```python
from build123d import *

# Parameters (mm, degrees)
SKETCH1_R           = 25
BOSS_EXTRUDE1_DEPTH = 40
CUT_EXTRUDE1_START  = -8
CUT_EXTRUDE1_DEPTH  = 8
CIRPATTERN1_COUNT   = 3
SKETCH7_R           = 15.1
CUT_EXTRUDE3_DEPTH  = 8.7
SKETCH8_R           = 1.5
CUT_EXTRUDE4_DEPTH  = 48.219593391


with BuildPart() as part:
    # Sketch1 → Boss-Extrude1 (new body)
    with BuildSketch(Plane(origin=(0, 0, 0), x_dir=(1, 0, 0), z_dir=(0, 1, 0))):
        with Locations(Location((0, 0, 0), (0, 0, 270))):
            Circle(SKETCH1_R)
    extrude(amount=BOSS_EXTRUDE1_DEPTH)

    # Sketch2 → Cut-Extrude1 (cut)
    with BuildSketch(Plane(origin=(0, 40, 0), x_dir=(1, 0, 0), z_dir=(0, 1, 0)).offset(CUT_EXTRUDE1_START)):
        with BuildLine():
            Line((-25, 0), (-5, 0))
            Line((-5, 0), (-5, -16.4))
            Line((-5, -16.4), (-13.2, -16.4))
            Line((-13.2, -16.4), (-13.2, -8.2))
            Line((-13.2, -8.2), (-23.616943071, -8.2))
            ThreePointArc((-23.616943071, -8.2), (-24.651811057, -4.157909525), (-25, 0))
        make_face()
    cut_extrude1 = extrude(amount=CUT_EXTRUDE1_DEPTH, mode=Mode.SUBTRACT)

    # CirPattern1: Cut-Extrude1 ×3 about axis
    cirpattern1_axis = Axis((0, 0, 0), (0, 1, 0))
    for i in range(1, CIRPATTERN1_COUNT):
        add(cut_extrude1.rotate(cirpattern1_axis, i * 360 / CIRPATTERN1_COUNT), mode=Mode.SUBTRACT)

    # Sketch7 → Cut-Extrude3 (cut)
    with BuildSketch(Plane.XZ):
        with Locations(Location((0, 0, 0), (0, 0, 270))):
            Circle(SKETCH7_R)
    extrude(amount=-CUT_EXTRUDE3_DEPTH, mode=Mode.SUBTRACT)

    # Sketch8 → Cut-Extrude4 (cut, through all)
    with BuildSketch(Plane.XZ.offset(-8.7)):
        with Locations(Location((0, 0, 0), (0, 0, 270))):
            Circle(SKETCH8_R)
    extrude(amount=-CUT_EXTRUDE4_DEPTH, mode=Mode.SUBTRACT)


solid = part.part
```
Here's how the part is built. I have some questions about the finished solid (model axes, mm). A direction names the side the tool comes from. Give positions to 0.01 mm unless a question says otherwise; leave off trailing zeros. Loops run counter-clockwise (first coordinate to the right, second up) from the corner with the lowest first, then second, coordinate; pieces in that order, holes last. Notation, with made-up numbers: M -22,63.25 L -17,63.25 A19 ccw -17,68.25 Z; hole C 68.25,52 d4. An arc over 180 degrees is marked long. Use one line per item in the form item = value. Start each with the question number.
Q1. Which directions (+Z, -Z, +X, -X, +Y, -Y) give clear straight access to the entire face, cutting with the end or side of a thin tool? Please do faces 5 (the flat face through (-18, 36, 8.2)), 6 (the flat face through (16.27, 35.94, 11.78)), 7 (the flat face through (0, 8.7, -3)), 8 (the flat face through (-9.7, 35.9, -16)).
Q2. If we section it at A-A (x = 10.5): Write out the boundary of the cut face in (y, z).
Q3. I need wall thicknesses on line 1 along X through (y, z) = (24, 0); line 2 along X through (y, z) = (5, 0); line 3 along Z through (x, y) = (0.5, 8.5) (3 decimals). Which ranges of each line are inside material? Lowest first, please.
Q4. If we section it at D-D (x = 20): Write out the boundary of the cut face in (y, z).
Q5. Will these pins go through, and if not, where does the flat tip stop? pin 1 Ø6 at (x, y) = (-15.5, 14.5) entering from +Z; pin 2 Ø6.5 at (y, z) = (37.5, 11.5) entering from +X; pin 3 Ø1.5 at (y, z) = (19, 2) entering from -X.
Q6. If we section it at B-B (y = 4): Write out the boundary of the cut face in (x, z), then the cut area to 3 significant figures.
Q7. Thinking about a two-plate mould opening in Z: for faces 1 (the cylindrical face through (7.509, 19.72, 23.846)), 2 (the flat face through (18.724, 35.944, -0.369)), 3 (the flat face through (-11, 0, 11)), 4 (the flat face through (2.066, 35.944, -19.979)), which applies, +Z half, -Z half, draft (parallel to the pull), parting line (faces both ways), or undercut?
Q8. If we section it at C-C (z = -14): Write out the boundary of the cut face in (x, y).
Taken from the geometry:
q1.face_5 = -X, +Y
q1.face_6 = +Z, +Y
q1.face_7 = -Y
q1.face_8 = +Y
q2.outline = M 0,-22.69 L 32,-22.69 L 32,-18.19 L 40,-18.19 L 40,-0.29 L 32,-0.29 L 32,18.19 L 40,18.19 L 40,22.69 L 0,22.69 L 0,10.85 L 8.7,10.85 L 8.7,-10.85 L 0,-10.85 Z
q3.line_1 = -25 to -1.5, 1.5 to 25
q3.line_2 = -25 to -15.1, 15.1 to 25
q3.line_3 = -24.995 to -15.092, 15.092 to 24.995
q4.outline = M 0,-15 L 40,-15 L 40,1.84 L 32,1.84 L 32,3.7 L 40,3.7 L 40,15 L 0,15 Z
q5.pin_1 = 21.65
q5.pin_2 = 23.6
q5.pin_3 = -24.97
q6.outline = C 0,0 d50; hole C 0,0 d30.2
q6.area = 1,250 mm^2
q7.face_1 = parting line
q7.face_2 = undercut
q7.face_3 = draft
q7.face_4 = undercut
q8.outline = M -20.71,0 L -5.66,0 L -5.66,8.7 L 5.66,8.7 L 5.66,0 L 20.71,0 L 20.71,40 L 8.08,40 L 8.08,32 L -10.85,32 L -10.85,40 L -20.71,40 Z
